```python
from build123d import *

# Parameters (mm, degrees)
F0_R     = 2.514559369
F1_DEPTH = 12
F1_TAPER = -5
F2_R     = 3
F4_D     = 3.3
F4_DEPTH = 9
F4_TIP   = 0.9914200214


with BuildPart() as f1:
    # F0 (on Top) → F1 (new body)
    with BuildSketch(Plane.XY):
        Circle(F0_R)
    extrude(amount=F1_DEPTH, taper=F1_TAPER)

    # F2
    f2_edges = [f1.edges().sort_by_distance(p)[0] for p in [
        (-3.564423, 0, 12),
    ]]
    fillet(f2_edges, radius=F2_R)

    # F4
    with Locations(Plane(origin=(0, 0, 0), x_dir=(1, 0, 0), z_dir=(0, 0, -1))):
        with Locations((0, 0)):
            Hole(F4_D / 2, depth=F4_DEPTH)
            with Locations((0, 0, -(F4_DEPTH + F4_TIP / 2))):  # 118° drill point
                Cone(0, F4_D / 2, F4_TIP, mode=Mode.SUBTRACT)


solid = f1.part
```
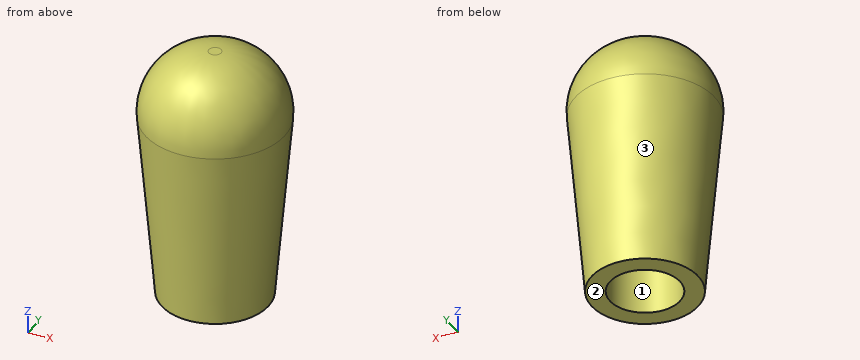
CAD build for the part. Positions are in the model's coordinates, mm. Face numbers are marked on the shaded views. Give positions to 0.01 mm unless a question says otherwise; leave off trailing zeros. Loops run counter-clockwise (first coordinate to the right, second up) from the corner with the lowest first, then second, coordinate; pieces in that order, holes last. Notation, with made-up numbers: M -33,-10 L -18,-10 A34 cw -18,26 Z; hole C 24,34.5 d2. An arc over 180 degrees is marked long. Use one line per item in the form item = value.
Item 1: Drill centre lines: probe 1 along X at (y, z) = (-0.75, 6.25); probe 2 along Y at (x, z) = (0, 5.25); probe 3 along Y at (x, z) = (-0.5, 1). Where is each one in solid material? Low to high. Write a range as from..to.
Determined:
probe_1 = -2.97..-1.47, 1.47..2.97
probe_2 = -2.97..-1.65, 1.65..2.97
probe_3 = -2.55..-1.57, 1.57..2.55
Item 2: Slice it at A-A (z = 4.25). List the corners of the cut face in (x, y), plus the area to 3 significant figures.
Determined:
outline = C 0,0 d5.77; hole C 0,0 d3.3
area = 17.6 mm2
Item 3: Flat gauge pins, fed straight in: pin 1 (3 mm diameter, centred on x = -0.5, z = 1.5, fed in from +Y); pin 2 (1.5 mm diameter, centred on x = 2, y = -2.5, fed in from -Z). Where does each tip first touch, or does it go through?
Determined:
pin_1 = 2.77
pin_2 = 0
Item 4: Slice it at B-B (z = 2.25). List the corners of the cut face in (x, y), plus the area to 3 significant figures.
Determined:
outline = C 0,0 d5.42; hole C 0,0 d3.3
area = 14.5 mm2
Item 5: Two-plate mould, pull along Y, no slides. Class the marked faces 1, 2 and 3: pulls with the +Y half, pulls with the -Y half, needs draft (parallel to the pull), parting line crosses it, or undercut.
Determined:
face_1 = undercut
face_2 = needs draft
face_3 = parting line crosses it
